Could you check a few things on this model? Use its own coordinates, in mm. A direction names the side the tool comes from. Coordinates: 2 decimals unless noted, no trailing zeros. Write each loop counter-clockwise with the first axis right and the second up, starting at its lowest first coordinate (ties: lowest second). Pieces come first, ordered by that corner, then holes. Notation, with made-up numbers: M 31,54.5 L 79,54.5 A24 cw 79,87.5 Z; hole C 17,69 d9. An arc over 180 degrees is marked long. Answer as CSV lines item,"result". Start each with the question number.
Item 1: We'd pull the mould along Z, two halves only. Please class faces 1 (the cylindrical face through (13.411, 9.367, -38.834)), 2 (the cylindrical face through (-16.589, 9.367, 31.166)), 3 (the flat face through (0, 0, -28)), 4 (the flat face through (0, 10, 45)): +Z half, -Z half, draft (parallel to the pull), parting line (faces both ways), or undercut.
Item 2: I'm going to push a flat-ended pin straight in: P1, Ø6.5, axis at x = -15, z = 35, coming from the +Y side. Where does the tip first touch, or does it pass through?
Item 3: Suppose I cut it at C-C, the plane x = -15. Write out the boundary of the cut face in (y, z) (3 decimals).
Item 4: On a 3-axis mill with a long thin cutter (end or side, diameter ignored), from which of +Z, -Z, +X, -X, +Y, -Y can I reach the whole of each face in a straight line? I mean faces 5 (the flat face through (0, 3, 10.125)), 6 (the cylindrical face through (13.411, 9.367, 31.166)). Say none if no direction works.
Item 5: Suppose I cut it at D-D, the plane x = 1. Write out the boundary of the cut face in (y, z) (3 decimals), and give its area (3 significant figures).
Item 6: Suppose I cut it at A-A, the plane z = 35. Write out the boundary of the cut face in (x, y).
Item 7: Suppose I cut it at B-B, the plane y = 8.5. Write out the boundary of the cut face in (x, z), and give its area (3 significant figures).
Item 8: If I drill on line 1 along X through (y, z) = (9.5, 35); line 2 along X through (y, z) = (6.25, 33); line 3 along Z through (x, y) = (-17.5, 2) (3 decimals), over which ranges is the centre line in solid material (lowest first)? Write a range as [from, to].
```python
from build123d import *

# Parameters (mm, degrees)
SKETCH1_W               = 50
SKETCH1_H               = 90
BOSS_EXTRUDE1_DEPTH     = 20
SKETCH2_W               = 20.25
SKETCH2_H               = 5.1
CUT_EXTRUDE1_DEPTH      = 1
CUT_EXTRUDE1_DEPTH_BACK = 51
SKETCH3_R               = 4.15
CUT_EXTRUDE2_DEPTH      = 21
CHAMFER1_SIZE           = 1
CHAMFER1_SIZE2          = 0.577350269
CHAMFER1_PART_2_SIZE    = 1
CHAMFER1_PART_2_SIZE2   = 0.577350269
CHAMFER1_PART_3_SIZE    = 1
CHAMFER1_PART_3_SIZE2   = 0.577350269
CHAMFER1_PART_4_SIZE    = 1
CHAMFER1_PART_4_SIZE2   = 0.577350269
CHAMFER2_SIZE           = 1


with BuildPart() as part:
    # Sketch1 → Boss-Extrude1 (new body)
    with BuildSketch(Plane(origin=(0, 0, 0), x_dir=(1, 0, 0), z_dir=(0, 1, 0))):
        Rectangle(SKETCH1_W, SKETCH1_H)
    extrude(amount=BOSS_EXTRUDE1_DEPTH)

    # Sketch2 → Cut-Extrude1 (cut, two sides)
    with BuildSketch(Plane(origin=(25, 0, 0), x_dir=(0, 0, -1), z_dir=(1, 0, 0))) as cut_extrude1_sk:
        with Locations((0, 2.55)):
            Rectangle(SKETCH2_W, SKETCH2_H)
    extrude(amount=CUT_EXTRUDE1_DEPTH, mode=Mode.SUBTRACT)
    extrude(cut_extrude1_sk.sketch, amount=-CUT_EXTRUDE1_DEPTH_BACK, mode=Mode.SUBTRACT)

    # Sketch3 → Cut-Extrude2 (cut, through all)
    with BuildSketch(Plane.XZ):
        with Locations(Location((-15, 35, 0), (0, 0, 270))):  # turned: the seam where the file's is
            Circle(SKETCH3_R)
        with Locations(Location((-15, -35, 0), (0, 0, 270))):  # turned: the seam where the file's is
            Circle(SKETCH3_R)
        with Locations(Location((15, 35, 0), (0, 0, 270))):  # turned: the seam where the file's is
            Circle(SKETCH3_R)
        with Locations(Location((15, -35, 0), (0, 0, 270))):  # turned: the seam where the file's is
            Circle(SKETCH3_R)
    extrude(amount=-CUT_EXTRUDE2_DEPTH, mode=Mode.SUBTRACT)

    # Chamfer1
    chamfer1_edges = [part.edges().sort_by_distance(p)[0] for p in [
        (-15, 20, 39.15),
    ]]
    chamfer1_side = [part.faces().sort_by_distance(p)[0] for p in [
        (-15, 10, 39.15),
    ]]
    chamfer(chamfer1_edges, length=CHAMFER1_SIZE, length2=CHAMFER1_SIZE2, reference=chamfer1_side[0])

    # Chamfer1 part 2
    chamfer1_part_2_edges = [part.edges().sort_by_distance(p)[0] for p in [
        (15, 20, 39.15),
    ]]
    chamfer1_part_2_side = [part.faces().sort_by_distance(p)[0] for p in [
        (15, 10, 39.15),
    ]]
    chamfer(chamfer1_part_2_edges, length=CHAMFER1_PART_2_SIZE, length2=CHAMFER1_PART_2_SIZE2, reference=chamfer1_part_2_side[0])

    # Chamfer1 part 3
    chamfer1_part_3_edges = [part.edges().sort_by_distance(p)[0] for p in [
        (15, 20, -30.85),
    ]]
    chamfer1_part_3_side = [part.faces().sort_by_distance(p)[0] for p in [
        (15, 10, -30.85),
    ]]
    chamfer(chamfer1_part_3_edges, length=CHAMFER1_PART_3_SIZE, length2=CHAMFER1_PART_3_SIZE2, reference=chamfer1_part_3_side[0])

    # Chamfer1 part 4
    chamfer1_part_4_edges = [part.edges().sort_by_distance(p)[0] for p in [
        (-15, 20, -30.85),
    ]]
    chamfer1_part_4_side = [part.faces().sort_by_distance(p)[0] for p in [
        (-15, 10, -30.85),
    ]]
    chamfer(chamfer1_part_4_edges, length=CHAMFER1_PART_4_SIZE, length2=CHAMFER1_PART_4_SIZE2, reference=chamfer1_part_4_side[0])

    # Chamfer2
    chamfer2_edges = [part.edges().sort_by_distance(p)[0] for p in [
        (0, 0, -10.125),
        (0, 0, 10.125),
    ]]
    chamfer(chamfer2_edges, length=CHAMFER2_SIZE)


solid = part.part
```
Ans:
1,face 1,"undercut"
1,face 2,"undercut"
1,face 3,"draft"
1,face 4,"+Z half"
2,P1,"passes through"
3,outline,"M 0,-45 L 20,-45 L 20,-39.727 L 19,-39.15 L 0,-39.15 Z; M 0,-30.85 L 19,-30.85 L 20,-30.273 L 20,30.273 L 19,30.85 L 0,30.85 L 0,11.125 L 1,10.125 L 5.1,10.125 L 5.1,-10.125 L 1,-10.125 L 0,-11.125 Z; M 0,39.15 L 19,39.15 L 20,39.727 L 20,45 L 0,45 Z"
4,face 5,"+X, -X, -Y"
4,face 6,"+Y, -Y"
5,outline,"M 0,-45 L 20,-45 L 20,45 L 0,45 L 0,11.125 L 1,10.125 L 5.1,10.125 L 5.1,-10.125 L 1,-10.125 L 0,-11.125 Z"
5,area,"1,700 mm^2"
6,outline,"M -25,0 L -19.15,0 L -19.15,19 L -19.73,20 L -25,20 Z; M -10.85,0 L 10.85,0 L 10.85,19 L 10.27,20 L -10.27,20 L -10.85,19 Z; M 19.15,0 L 25,0 L 25,20 L 19.73,20 L 19.15,19 Z"
7,outline,"M -25,-45 L 25,-45 L 25,45 L -25,45 Z; hole C -15,-35 d8.3; hole C -15,35 d8.3; hole C 15,-35 d8.3; hole C 15,35 d8.3"
7,area,"4,280 mm^2"
8,line 1,"x = [-25, -19.15], [-10.85, 10.85], [19.15, 25]"
8,line 2,"x = [-25, -18.64], [-11.36, 11.36], [18.64, 25]"
8,line 3,"z = [-45, -38.312], [-31.688, -10.125], [10.125, 31.688], [38.312, 45]"
